```python
from build123d import *

# Parameters (mm, degrees)
SKETCH_R        = 34
SKETCH_R_2      = 31
PAD_DEPTH       = 10
SKETCH001_R     = 32.5
POCKET_DEPTH    = 7
SKETCH002_R     = 32.5
POCKET001_DEPTH = 1.25


with BuildPart() as part:
    # Sketch → Pad (new body)
    with BuildSketch(Plane.XY):
        Circle(SKETCH_R)
        Circle(SKETCH_R_2, mode=Mode.SUBTRACT)
    extrude(amount=PAD_DEPTH)

    # Sketch001 → Pocket (cut)
    with BuildSketch(Plane.XY):
        Circle(SKETCH001_R)
    extrude(amount=POCKET_DEPTH, mode=Mode.SUBTRACT)

    # Sketch002 → Pocket001 (cut)
    with BuildSketch(Plane.XY.offset(10)):
        Circle(SKETCH002_R)
    extrude(amount=-POCKET001_DEPTH, mode=Mode.SUBTRACT)


solid = part.part
```
Geometry check sheet. Reference: the model listing, model coordinates, mm. A direction names the side the tool comes from. Round coordinates to 2 decimals unless told otherwise and drop trailing zeros. Loops run counter-clockwise (first coordinate to the right, second up) from the corner with the lowest first, then second, coordinate; pieces in that order, holes last. Notation, with made-up numbers: (54.25, 62.5) - (98.25, 62.5) arc R31 ccw to (98.25, 87.5) - close; hole circle Ø1 at (-23, 60). An arc over 180 degrees is marked (long way). Write item = value, one per line. Start each with the question number.
1. Thickness scan on line 1 (Y direction, x = 0, z = 9.5); line 2 (Y direction, x = 0, z = 7.45); line 3 (X direction, y = 28.5, z = 4.25). Record the ranges inside material, lowest first.
2. Set-up check for faces 1 (the face through (29, -12, 8.75)), 2 (the face through (28, -17, 0)), 3 (the face through (31, 9.76, 3.45)): record each of +Z, -Z, +X, -X, +Y, -Y from which the full face is reachable in a straight line by a thin tool's end or side.
3. Depth check by flat-ended pin: pin 1 (3 mm diameter, centred on y = 21, z = 2.5, fed in from +X); pin 2 (1 mm diameter, centred on y = -9, z = 6, fed in from -X); pin 3 (5 mm diameter, centred on x = 13.5, y = -24, fed in from +Z); pin 4 (6 mm diameter, centred on x = 10, z = 7.5, fed in from +Y). Enter the tip coordinate at first touch or a pass-through.
4. Mould release check, pull along Y, two halves, no side actions. Record for faces 4 (the face through (18.28, 28.67, 4.93)), 5 (the face through (28, -17, 10)), 6 (the face through (29, -12, 7)), 7 (the face through (31, 9.76, 9.38)): released by +Y, released by -Y, zero draft, split by the parting line, or undercut.
5. Section check C-C on z = 6. Enter the section's corners in (x, y), then the cut area to 3 significant figures.
6. Section check A-A on y = 0. Enter the section's corners in (x, z).
Working result:
q1.line_1 = -34 to -32.5, 32.5 to 34
q1.line_2 = -34 to -31, 31 to 34
q1.line_3 = -18.54 to -15.62, 15.62 to 18.54
q2.face_1 = +Z
q2.face_2 = -Z, +X, -X, +Y, -Y
q2.face_3 = -Z
q3.pin_1 = 27.85
q3.pin_2 = -32.92
q3.pin_3 = through
q3.pin_4 = 33.27
q4.face_4 = split by the parting line
q4.face_5 = zero draft
q4.face_6 = undercut
q4.face_7 = undercut
q5.outline = circle Ø68 at (0, 0); hole circle Ø65 at (0, 0)
q5.area = 313 mm^2
q6.outline = (-34, 0) - (-32.5, 0) - (-32.5, 7) - (-31, 7) - (-31, 8.75) - (-32.5, 8.75) - (-32.5, 10) - (-34, 10) - close; (31, 7) - (32.5, 7) - (32.5, 0) - (34, 0) - (34, 10) - (32.5, 10) - (32.5, 8.75) - (31, 8.75) - close
